from build123d import *

# Parameters (mm, degrees)
F0_W     = 50.8
F0_H     = 38.1
F1_DEPTH = 25.4
F3_DEPTH = 12.7
F5_DEPTH = 25.4


with BuildPart() as f1:
    # F0 (on Top) → F1 (new body)
    with BuildSketch(Plane.XY):
        with Locations((65.2933099031, -40.0903208673)):
            Rectangle(F0_W, F0_H)
    extrude(amount=F1_DEPTH)

    # F2 (on face) → F3 (cut)
    with BuildSketch(Plane.XY.offset(25.4)):
        Polygon((90.6933099031, -21.0403208673), (52.5933099031, -21.0403208673), (71.6433099031, -59.1403208673), (90.6933099031, -59.1403208673), align=None)
    extrude(amount=-F3_DEPTH, mode=Mode.SUBTRACT)

    # F4 (on face) → F5 (cut)
    with BuildSketch(Plane.XY.offset(12.7)):
        Polygon((90.6933099031, -21.0403208673), (77.9933099031, -21.0403208673), (90.6933099031, -40.0903208673), align=None)
    extrude(amount=-F5_DEPTH, mode=Mode.SUBTRACT)


solid = f1.part
Build history of the part. All positions in model axes, mm. A direction names the side the tool comes from. Coordinates: 2 decimals unless noted, no trailing zeros. Order: outer loops, then holes, each group sorted by start corner. A loop starts at its lowest first (then second) coordinate and runs counter-clockwise, first axis right, second up. Notation, with made-up numbers: (5, 15) - (55, 15) arc R10 cw to (55, 21) - close; hole circle Ø2 at (50.5, -30.75). An arc over 180 degrees is marked (long way). Write each question's results on one line, items separated by ' | '. Start each with the question number.
Item 1: Band-saw the part on C-C on y = -42.5. Write the cut outline in (x, z), and give its area (3 significant figures).
Item 2: Flat gauge pins, fed straight in: pin 1 (2 mm diameter, centred on y = -26, z = 6.5, fed in from +X); pin 2 (5 mm diameter, centred on x = 67, y = -30.5, fed in from +Z). Where does each tip first touch, or does it go through?
Item 3: Band-saw the part on D-D on y = -31. Write the cut outline in (x, z).
Item 4: Band-saw the part on B-B on x = 75. Write the cut outline in (y, z).
Item 5: Band-saw the part on A-A on z = 2. Write the cut outline in (x, y), and give its area (3 significant figures).
Item 6: Wall check: probe 1 along Z at (x, y) = (65, -35.5); probe 2 along X at (y, z) = (-49, 21); probe 3 along Y at (x, z) = (81, 2.5). Give the ranges that are in metal, low to high. Write a range as [from, to].
Item 7: Tool access for faces 1 (the face through (59, -59.14, 13)), 2 (the face through (61.985, -39.824, 19.139)): list every direction of +Z, -Z, +X, -X, +Y, -Y with a clear straight run to the whole face (end or side of a thin tool).
Numbers:
1) outline: (39.89, 0) - (90.69, 0) - (90.69, 12.7) - (63.32, 12.7) - (63.32, 25.4) - (39.89, 25.4) - close | area: 943 mm^2
2) pin 1: x = 81.97 | pin 2: z = 12.7
3) outline: (39.89, 0) - (84.63, 0) - (84.63, 12.7) - (57.57, 12.7) - (57.57, 25.4) - (39.89, 25.4) - close
4) outline: (-59.14, 0) - (-21.04, 0) - (-21.04, 12.7) - (-59.14, 12.7) - close
5) outline: (39.89, -59.14) - (90.69, -59.14) - (90.69, -40.09) - (77.99, -21.04) - (39.89, -21.04) - close | area: 1,810 mm^2
6) probe 1: [0, 12.7] | probe 2: [39.89, 66.57] | probe 3: [-59.14, -25.55]
7) face 1: +Z, -Z, +X, -X, -Y | face 2: +Z, +X, +Y
